Geometry check sheet. Reference: the model listing, model coordinates, mm. Face numbers are marked on the shaded views. A direction names the side the tool comes from. Give positions to 0.01 mm unless a question says otherwise; leave off trailing zeros. Write each loop counter-clockwise with the first axis right and the second up, starting at its lowest first coordinate (ties: lowest second). Pieces come first, ordered by that corner, then holes. Notation, with made-up numbers: (38.25, 4.25) -> (43.25, 4.25) arc R23 ccw to (43.25, 19.25) -> close; hole circle Ø11 at (-8.5, 3). An arc over 180 degrees is marked (long way). Use a Markdown table: item, result. Add a question column.
from build123d import *

# Parameters (mm, degrees)
CYLINDER001_R     = 1.6
CYLINDER001_DEPTH = 5
BOX001_W          = 27
BOX001_H          = 5
BOX001_DEPTH      = 9
FILLET_R          = 3
BOX002_W          = 4
BOX002_H          = 8
BOX002_DEPTH      = 12
FILLET002_R       = 2
CYLINDER_R        = 2.8
CYLINDER_DEPTH    = 2
BOX_W             = 27
BOX_H             = 2
BOX_DEPTH         = 9
FILLET001_R       = 3


with BuildPart() as screw_hole:
    # Cylinder001 → Cylinder001 (new body)
    with BuildSketch(Plane(origin=(22.2, 3, 4.5), x_dir=(1, 0, 0), z_dir=(0, 1, 0))):
        Circle(CYLINDER001_R)
    extrude(amount=CYLINDER001_DEPTH)


with BuildPart() as back_cut:
    # Box001 → Box001 (new body)
    with BuildSketch(Plane(origin=(0, 3, 0), x_dir=(1, 0, 0), z_dir=(0, 0, 1))):
        with Locations((13.5, 2.5)):
            Rectangle(BOX001_W, BOX001_H)
    extrude(amount=BOX001_DEPTH)

    # Fillet
    fillet_edges = [back_cut.edges().sort_by_distance(p)[0] for p in [
        (27, 5.5, 9),
        (27, 5.5, 0),
    ]]
    fillet(fillet_edges, radius=FILLET_R)

    # Cut001: cut screw hole
    add(screw_hole.part, mode=Mode.SUBTRACT)


with BuildPart() as glue_cube_fillet:
    # Box002 → Box002 (new body)
    with BuildSketch(Plane.XY):
        with Locations((2, 4)):
            Rectangle(BOX002_W, BOX002_H)
    extrude(amount=BOX002_DEPTH)

    # Fillet002
    fillet002_edges = [glue_cube_fillet.edges().sort_by_distance(p)[0] for p in [
        (2, 0, 12),
        (2, 8, 12),
    ]]
    fillet(fillet002_edges, radius=FILLET002_R)


with BuildPart() as pass_hole:
    # Cylinder → Cylinder (new body)
    with BuildSketch(Plane(origin=(22.2, 0, 4.5), x_dir=(1, 0, 0), z_dir=(0, 1, 0))):
        Circle(CYLINDER_R)
    extrude(amount=CYLINDER_DEPTH)


with BuildPart() as power_socket_screw_connector:
    # Box → Box (new body)
    with BuildSketch(Plane.XY):
        with Locations((13.5, 1)):
            Rectangle(BOX_W, BOX_H)
    extrude(amount=BOX_DEPTH)

    # Fillet001
    fillet001_edges = [power_socket_screw_connector.edges().sort_by_distance(p)[0] for p in [
        (27, 1, 9),
        (27, 1, 0),
    ]]
    fillet(fillet001_edges, radius=FILLET001_R)

    # Cut: cut pass hole
    add(pass_hole.part, mode=Mode.SUBTRACT)

    # Fusion: union back cut, glue cube fillet
    add(back_cut.part)
    add(glue_cube_fillet.part)


solid = power_socket_screw_connector.part
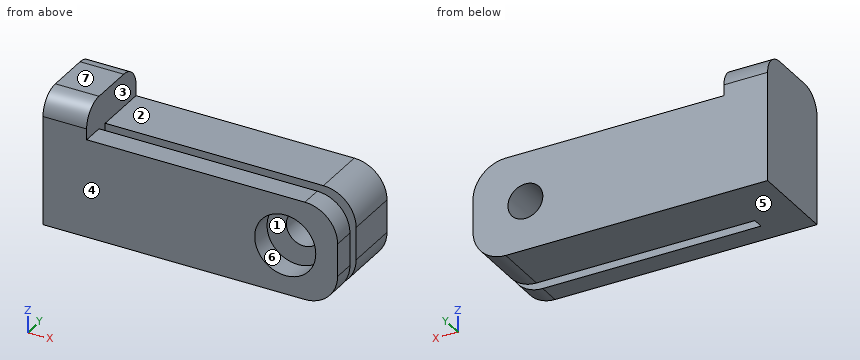
1) Material ranges on probe 1 along Y at (x, z) = (11.75, 5); probe 2 along Z at (x, y) = (22.2, 5.7); probe 3 along X at (y, z) = (5.7, 4.5), recorded low to high. Write a range as [from, to].
2) Sectioned sample at A-A, the plane z = 4.5. Enter the section's corners in (x, y), and give its area (3 significant figures).
3) Draft check along Z on the marked faces 5, 6 and 7. Enter one of: +Z half, -Z half, draft (parallel to the pull), parting line (faces both ways), or undercut.
4) Tool access check on the marked faces 1, 2, 3 and 4. Record the directions out of +Z, -Z, +X, -X, +Y, -Y that give a thin tool (end or side, any length) a straight path to the whole face; none if there is none.
5) Gauge pin test, flat ends, axial feed: P1, Ø5, axis at x = 22.2, z = 4.5, coming from the -Y side; P2, Ø2.5, axis at x = 22.2, z = 4.5, coming from the +Y side; P3, Ø1, axis at x = 17, y = 1, coming from the +Z side. Record the tip position at first contact, or that the pin passes through.
6) Sectioned sample at D-D, the plane x = 22.2. Enter the section's corners in (y, z).
7) Sectioned sample at C-C, the plane x = 13.75. Enter the section's corners in (y, z), and give its area (3 significant figures).
8) Sectioned sample at B-B, the plane y = 5.5. Enter the section's corners in (x, z).
Check values:
| question | item | result |
|---|---|---|
| 1 | probe 1 | [0, 2], [3, 8] |
| 1 | probe 2 | [0, 2.9], [6.1, 9] |
| 1 | probe 3 | [0, 20.6], [23.8, 27] |
| 2 | outline | (0, 0) -> (19.4, 0) -> (19.4, 2) -> (4, 2) -> (4, 3) -> (20.6, 3) -> (20.6, 8) -> (0, 8) -> close; (23.8, 3) -> (27, 3) -> (27, 8) -> (23.8, 8) -> close; (25, 0) -> (27, 0) -> (27, 2) -> (25, 2) -> close |
| 2 | area | 166 mm² |
| 3 | face 5 | -Z half |
| 3 | face 6 | undercut |
| 3 | face 7 | +Z half |
| 4 | face 1 | +Z, -Z, +X |
| 4 | face 2 | +Z, +X, +Y, -Y |
| 4 | face 3 | +Z, +X |
| 4 | face 4 | +Z, -Z, +X, -X, -Y |
| 5 | P1 | y = 3 |
| 5 | P2 | through |
| 5 | P3 | z = 9 |
| 6 | outline | (0, 0) -> (2, 0) -> (2, 1.7) -> (0, 1.7) -> close; (0, 7.3) -> (2, 7.3) -> (2, 9) -> (0, 9) -> close; (3, 0) -> (8, 0) -> (8, 2.9) -> (3, 2.9) -> close; (3, 6.1) -> (8, 6.1) -> (8, 9) -> (3, 9) -> close |
| 7 | outline | (0, 0) -> (2, 0) -> (2, 9) -> (0, 9) -> close; (3, 0) -> (8, 0) -> (8, 9) -> (3, 9) -> close |
| 7 | area | 63.0 mm² |
| 8 | outline | (0, 0) -> (24, 0) arc R3 ccw to (27, 3) -> (27, 6) arc R3 ccw to (24, 9) -> (4, 9) -> (4, 12) -> (0, 12) -> close; hole circle Ø3.2 at (22.2, 4.5) |
